Geometry: final body of the model. Coordinates: model frame, mm. Face numbers are marked on the shaded views. A direction names the side the tool comes from. Give positions to 0.01 mm unless a question says otherwise; leave off trailing zeros. Order: outer loops, then holes, each group sorted by start corner. A loop starts at its lowest first (then second) coordinate and runs counter-clockwise, first axis right, second up. Notation, with made-up numbers: M 30.25,75.5 L 65.25,75.5 A11 cw 65.25,92.5 Z; hole C -13,33.25 d8. An arc over 180 degrees is marked long. Use CSV: the item, a comma, the result in double quotes.
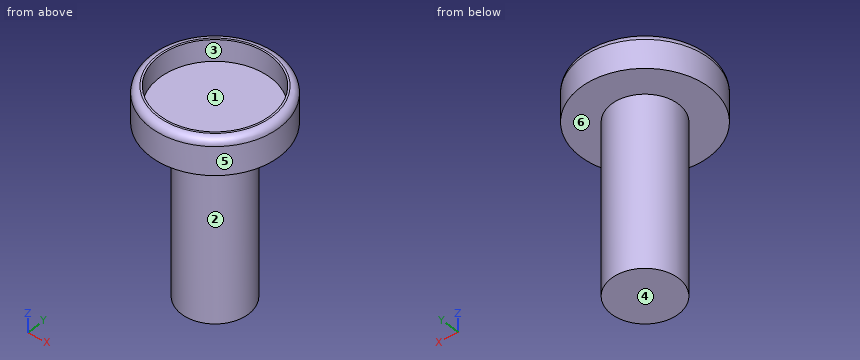
```python
from build123d import *

# Parameters (mm, degrees)
F0_R     = 4.675
F1_DEPTH = 24
F2_R     = 9
F3_DEPTH = 5
F4_R     = 7.75
F5_DEPTH = 3
F6_R     = 1


with BuildPart() as f1:
    # F0 (on Top) → F1 (new body)
    with BuildSketch(Plane.XY):
        Circle(F0_R)
    extrude(amount=F1_DEPTH)

    # F2 (on face) → F3 (join)
    with BuildSketch(Plane.XY.offset(24)):
        Circle(F2_R)
    extrude(amount=F3_DEPTH)

    # F4 (on face) → F5 (cut)
    with BuildSketch(Plane.XY.offset(29)):
        Circle(F4_R)
    extrude(amount=-F5_DEPTH, mode=Mode.SUBTRACT)

    # F6
    f6_edges = [f1.edges().sort_by_distance(p)[0] for p in [
        (-9, 0, 29),
    ]]
    fillet(f6_edges, radius=F6_R)


solid = f1.part
```
1. Pin query (flat end, axial travel): pin 1 Ø1 at (x, z) = (1, 13) entering from +Y; pin 2 Ø3 at (x, y) = (-2.5, 1) entering from +Z; pin 3 Ø4 at (x, y) = (3.5, 6.5) entering from -Z; pin 4 Ø8 at (x, y) = (-2, 3.5) entering from +Z. Return the tip coordinate at first contact, or that it passes through.
Answer:
pin 1,"y = 4.65"
pin 2,"z = 26"
pin 3,"z = 24"
pin 4,"z = 29"
2. Line query: line 1 (Y direction, x = 0, z = 28); line 2 (Z direction, x = -3.75, y = 1.5); line 3 (Z direction, x = 7, y = 0.75). Output: solid intervals per line, ascending.
Answer:
line 1,"-9 to -7.75, 7.75 to 9"
line 2,"0 to 26"
line 3,"24 to 26"
3. Reachability of the marked faces 5 and 6 from +Z, -Z, +X, -X, +Y, -Y: full face, straight path, thin tool, end or side. Return the list, or none.
Answer:
face 5,"+Z, -Z"
face 6,"-Z"
4. Section C-C, the plane z = 2.5. Return the cut outline in (x, y) (3 decimals), plus the area to 3 significant figures.
Answer:
outline,"C 0,0 d9.35"
area,"68.7 mm2"
5. Pull-direction query (Y, two-part tool) for the marked faces 1, 2, 3 and 4; classes: +Y half, -Y half, draft (parallel to the pull), parting line (faces both ways), or undercut.
Answer:
face 1,"undercut"
face 2,"parting line"
face 3,"undercut"
face 4,"draft"
6. Section A-A, the plane y = 0. Return the cut outline in (x, z) (3 decimals), plus the area to 3 significant figures.
Answer:
outline,"M -9,24 L -4.675,24 L -4.675,0 L 4.675,0 L 4.675,24 L 9,24 L 9,28 A1 ccw 8,29 L 7.75,29 L 7.75,26 L -7.75,26 L -7.75,29 L -8,29 A1 ccw -9,28 Z"
area,"267 mm2"
